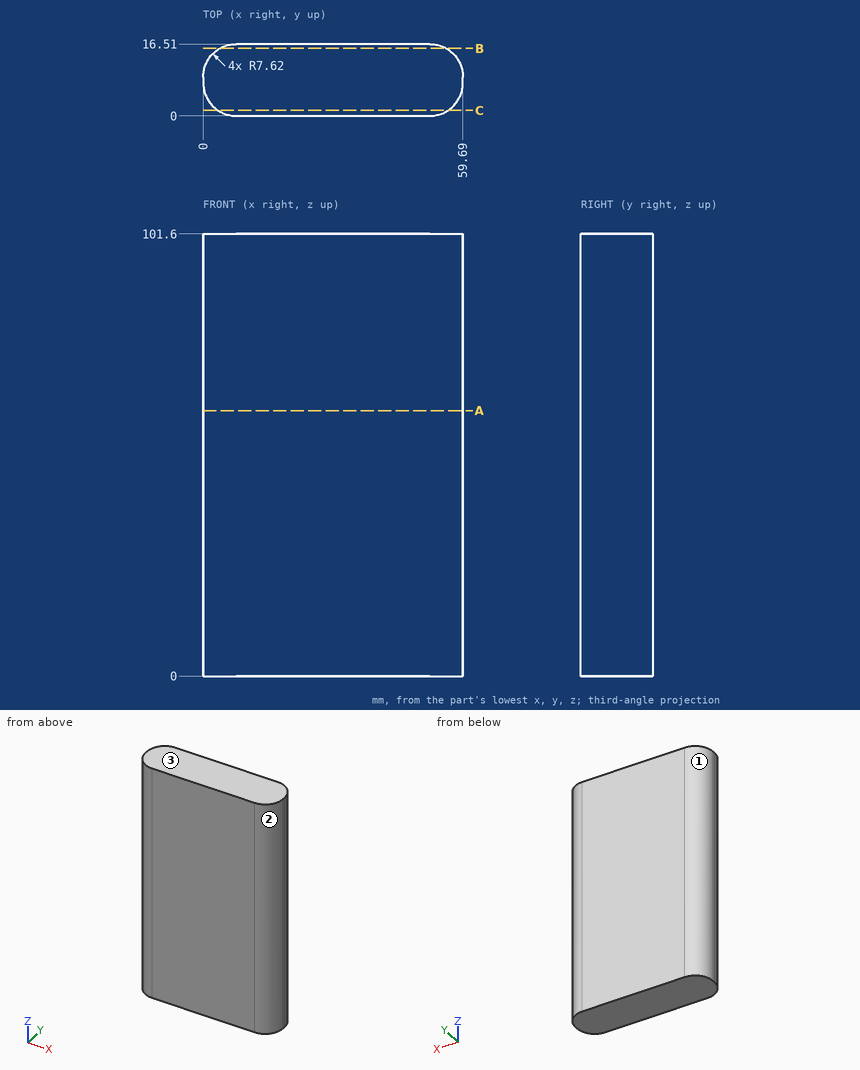
Input: dimensioned drawing with shaded views. Units: mm. Origin: part minimum x, y, z. Round coordinates to 2 decimals unless told otherwise and drop trailing zeros. Order: outer loops, then holes, each group sorted by start corner. A loop starts at its lowest first (then second) coordinate and runs counter-clockwise, first axis right, second up.
Q1. Mould query, pull axis X, two halves, no side actions, for the marked faces 1, 2 and 3. Classes: released by +X, released by -X, zero draft, split by the parting line, or undercut.
Result sheet:
face 1: released by -X
face 2: released by +X
face 3: zero draft
Q2. Pin query (flat end, axial travel): pin 1 (1.5 mm diameter, centred on y = 6.5, z = 62.5, fed in from +X); pin 2 (1.5 mm diameter, centred on y = 4.5, z = 36.5, fed in from +X). Return the tip coordinate at first contact, or that it passes through.
Result sheet:
pin 1: stops at x = 59.68
pin 2: stops at x = 59.31
Q3. Material intervals for probe 1 along X at (y, z) = (15.5, 90); probe 2 along X at (y, z) = (4.25, 24); probe 3 along Y at (x, z) = (57.5, 90), sorted ascending.
Result sheet:
probe 1: x = 3.83 to 55.86
probe 2: x = 0.79 to 58.9
probe 3: y = 2.27 to 14.24
Q4. Section A-A, the plane z = 61. Output: boundary loops of the cut face in (x, y), and give its area (3 significant figures).
Result sheet:
outline: (0, 7.62) arc R7.62 ccw to (7.62, 0) - (52.07, 0) arc R7.62 ccw to (59.69, 7.62) - (59.69, 8.89) arc R7.62 ccw to (52.07, 16.51) - (7.62, 16.51) arc R7.62 ccw to (0, 8.89) - close
area: 936 mm2
Q5. Section B-B, the plane y = 15.5. Output: boundary loops of the cut face in (x, z).
Result sheet:
outline: (3.83, 0) - (55.86, 0) - (55.86, 101.6) - (3.83, 101.6) - close
Q6. Section C-C, the plane y = 1.25. Output: boundary loops of the cut face in (x, z), and give its area (3 significant figures).
Result sheet:
outline: (3.44, 0) - (56.25, 0) - (56.25, 101.6) - (3.44, 101.6) - close
area: 5,370 mm2
